Geometry check sheet. Reference: the model listing, model coordinates, mm. Give positions to 0.01 mm unless a question says otherwise; leave off trailing zeros. Loops run counter-clockwise (first coordinate to the right, second up) from the corner with the lowest first, then second, coordinate; pieces in that order, holes last. Notation, with made-up numbers: (7, 74.25) -> (32, 74.25) arc R29 ccw to (32, 113.25) -> close; hole circle Ø6 at (-22.5, -20.5). An arc over 180 degrees is marked (long way). Write item = value, one per line. Start each with the question number.
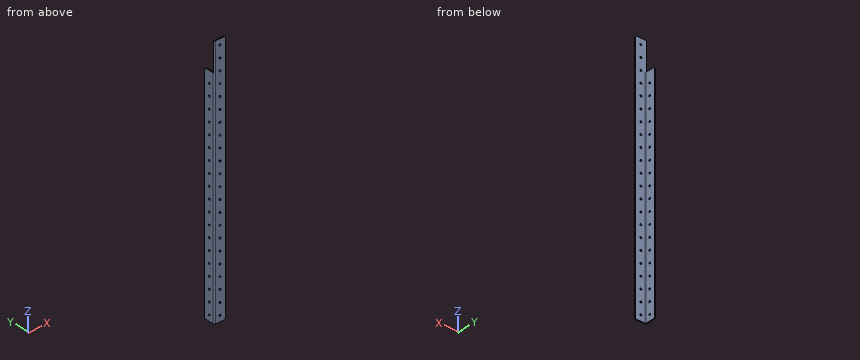
```python
from build123d import *

# Parameters (mm, degrees)
CUT_EXTRUDE1_OUTLINE_R   = 2.0701
CUT_EXTRUDE1_DEPTH       = 3.0988
CUT_EXTRUDE1_START       = 2.286
CUT_EXTRUDE1_2_OUTLINE_W = 2.286
CUT_EXTRUDE1_2_OUTLINE_H = 558.8
CUT_EXTRUDE1_2_DEPTH     = 23.114
CUT_EXTRUDE1_START_2     = 3.0988
CUT_EXTRUDE1_3_OUTLINE_W = 0.8128
CUT_EXTRUDE1_3_OUTLINE_H = 558.8
CUT_EXTRUDE1_3_DEPTH     = 22.3012
CUT_EXTRUDE1_4_OUTLINE_R = 2.0701
CUT_EXTRUDE1_4_DEPTH     = 2.286
CUT_EXTRUDE1_START_3     = -749.3
CUT_EXTRUDE1_5_DEPTH     = 558.8
CUT_EXTRUDE1_START_4     = 546.268979845
CUT_EXTRUDE1_6_OUTLINE_W = 4
CUT_EXTRUDE1_6_OUTLINE_H = 359
CUT_EXTRUDE1_6_DEPTH     = 2.731020155
CHAMFER1_SIZE            = 2.159
CUT_EXTRUDE2_START       = -2.286
SKETCH2_W                = 63.5
SKETCH2_H                = 23.114
CUT_EXTRUDE2_DEPTH       = 3.0988
CHAMFER2_SIZE            = 2.159
BOSS_EXTRUDE1_START      = -2.286
BOSS_EXTRUDE1_DEPTH      = 2.286


with BuildPart() as part:
    # Cut-Extrude1: read off the stored shape, not the designer's step
    # Cut-Extrude1 outline → Cut-Extrude1 (new body)
    with BuildSketch(Plane(origin=(0, 0, 0), x_dir=(1, 0, 0), z_dir=(0, 1, 0))):
        Polygon((0, 749.3), (0, 190.5), (25.4, 190.5), (25.4, 747.141), (23.241, 749.3), align=None)
        with Locations((12.7, 736.6)):
            Circle(CUT_EXTRUDE1_OUTLINE_R, mode=Mode.SUBTRACT)
        with Locations((12.7, 203.2)):
            Circle(CUT_EXTRUDE1_OUTLINE_R, mode=Mode.SUBTRACT)
        with Locations((12.7, 228.6)):
            Circle(CUT_EXTRUDE1_OUTLINE_R, mode=Mode.SUBTRACT)
        with Locations((12.7, 254)):
            Circle(CUT_EXTRUDE1_OUTLINE_R, mode=Mode.SUBTRACT)
        with Locations((12.7, 279.4)):
            Circle(CUT_EXTRUDE1_OUTLINE_R, mode=Mode.SUBTRACT)
        with Locations((12.7, 304.8)):
            Circle(CUT_EXTRUDE1_OUTLINE_R, mode=Mode.SUBTRACT)
        with Locations((12.7, 330.2)):
            Circle(CUT_EXTRUDE1_OUTLINE_R, mode=Mode.SUBTRACT)
        with Locations((12.7, 355.6)):
            Circle(CUT_EXTRUDE1_OUTLINE_R, mode=Mode.SUBTRACT)
        with Locations((12.7, 381)):
            Circle(CUT_EXTRUDE1_OUTLINE_R, mode=Mode.SUBTRACT)
        with Locations((12.7, 406.4)):
            Circle(CUT_EXTRUDE1_OUTLINE_R, mode=Mode.SUBTRACT)
        with Locations((12.7, 431.8)):
            Circle(CUT_EXTRUDE1_OUTLINE_R, mode=Mode.SUBTRACT)
        with Locations((12.7, 457.2)):
            Circle(CUT_EXTRUDE1_OUTLINE_R, mode=Mode.SUBTRACT)
        with Locations((12.7, 482.6)):
            Circle(CUT_EXTRUDE1_OUTLINE_R, mode=Mode.SUBTRACT)
        with Locations((12.7, 508)):
            Circle(CUT_EXTRUDE1_OUTLINE_R, mode=Mode.SUBTRACT)
        with Locations((12.7, 533.4)):
            Circle(CUT_EXTRUDE1_OUTLINE_R, mode=Mode.SUBTRACT)
        with Locations((12.7, 558.8)):
            Circle(CUT_EXTRUDE1_OUTLINE_R, mode=Mode.SUBTRACT)
        with Locations((12.7, 584.2)):
            Circle(CUT_EXTRUDE1_OUTLINE_R, mode=Mode.SUBTRACT)
        with Locations((12.7, 609.6)):
            Circle(CUT_EXTRUDE1_OUTLINE_R, mode=Mode.SUBTRACT)
        with Locations((12.7, 635)):
            Circle(CUT_EXTRUDE1_OUTLINE_R, mode=Mode.SUBTRACT)
        with Locations((12.7, 660.4)):
            Circle(CUT_EXTRUDE1_OUTLINE_R, mode=Mode.SUBTRACT)
        with Locations((12.7, 685.8)):
            Circle(CUT_EXTRUDE1_OUTLINE_R, mode=Mode.SUBTRACT)
        with Locations((12.7, 711.2)):
            Circle(CUT_EXTRUDE1_OUTLINE_R, mode=Mode.SUBTRACT)
    extrude(amount=CUT_EXTRUDE1_DEPTH)

    # Cut-Extrude1 2 outline → Cut-Extrude1 2 (add)
    with BuildSketch(Plane(origin=(0, 0, 0), x_dir=(1, 0, 0), z_dir=(0, 1, 0)).offset(CUT_EXTRUDE1_START)):
        with Locations((1.143, 469.9)):
            Rectangle(CUT_EXTRUDE1_2_OUTLINE_W, CUT_EXTRUDE1_2_OUTLINE_H)
    extrude(amount=CUT_EXTRUDE1_2_DEPTH)

    # Cut-Extrude1 3 outline → Cut-Extrude1 3 (cut)
    with BuildSketch(Plane.YZ.offset(CUT_EXTRUDE1_START_2)):
        with Locations((2.6924, -469.9)):
            Rectangle(CUT_EXTRUDE1_3_OUTLINE_W, CUT_EXTRUDE1_3_OUTLINE_H)
    extrude(amount=CUT_EXTRUDE1_3_DEPTH, mode=Mode.SUBTRACT)

    # Cut-Extrude1 4 outline → Cut-Extrude1 4 (cut)
    with BuildSketch(Plane.YZ):
        with Locations((12.7, -736.6)):
            Circle(CUT_EXTRUDE1_4_OUTLINE_R)
        with Locations((12.7, -711.2)):
            Circle(CUT_EXTRUDE1_4_OUTLINE_R)
        with Locations((12.7, -685.8)):
            Circle(CUT_EXTRUDE1_4_OUTLINE_R)
        with Locations((12.7, -660.4)):
            Circle(CUT_EXTRUDE1_4_OUTLINE_R)
        with Locations((12.7, -635)):
            Circle(CUT_EXTRUDE1_4_OUTLINE_R)
        with Locations((12.7, -609.6)):
            Circle(CUT_EXTRUDE1_4_OUTLINE_R)
        with Locations((12.7, -584.2)):
            Circle(CUT_EXTRUDE1_4_OUTLINE_R)
        with Locations((12.7, -558.8)):
            Circle(CUT_EXTRUDE1_4_OUTLINE_R)
        with Locations((12.7, -533.4)):
            Circle(CUT_EXTRUDE1_4_OUTLINE_R)
        with Locations((12.7, -508)):
            Circle(CUT_EXTRUDE1_4_OUTLINE_R)
        with Locations((12.7, -482.6)):
            Circle(CUT_EXTRUDE1_4_OUTLINE_R)
        with Locations((12.7, -457.2)):
            Circle(CUT_EXTRUDE1_4_OUTLINE_R)
        with Locations((12.7, -431.8)):
            Circle(CUT_EXTRUDE1_4_OUTLINE_R)
        with Locations((12.7, -406.4)):
            Circle(CUT_EXTRUDE1_4_OUTLINE_R)
        with Locations((12.7, -381)):
            Circle(CUT_EXTRUDE1_4_OUTLINE_R)
        with Locations((12.7, -355.6)):
            Circle(CUT_EXTRUDE1_4_OUTLINE_R)
        with Locations((12.7, -330.2)):
            Circle(CUT_EXTRUDE1_4_OUTLINE_R)
        with Locations((12.7, -304.8)):
            Circle(CUT_EXTRUDE1_4_OUTLINE_R)
        with Locations((12.7, -279.4)):
            Circle(CUT_EXTRUDE1_4_OUTLINE_R)
        with Locations((12.7, -254)):
            Circle(CUT_EXTRUDE1_4_OUTLINE_R)
        with Locations((12.7, -228.6)):
            Circle(CUT_EXTRUDE1_4_OUTLINE_R)
        with Locations((12.7, -203.2)):
            Circle(CUT_EXTRUDE1_4_OUTLINE_R)
    extrude(amount=CUT_EXTRUDE1_4_DEPTH, mode=Mode.SUBTRACT)

    # Cut-Extrude1 5 outline → Cut-Extrude1 5 (cut)
    with BuildSketch(Plane.XY.offset(CUT_EXTRUDE1_START_3)):
        with BuildLine():
            ThreePointArc((3.0988, 0), (0.907617506, 0.907617506), (0, 3.0988))
            Line((0, 3.0988), (0, 0))
            Line((0, 0), (3.0988, 0))
        make_face()
        with BuildLine():
            Line((3.0988, 3.0988), (2.286, 3.0988))
            ThreePointArc((2.286, 3.0988), (2.524063608, 2.524063608), (3.0988, 2.286))
            Line((3.0988, 2.286), (3.0988, 3.0988))
        make_face()
    extrude(amount=CUT_EXTRUDE1_5_DEPTH, mode=Mode.SUBTRACT)

    # Cut-Extrude1 6 outline → Cut-Extrude1 6 (cut)
    with BuildSketch(Plane(origin=(0, 0, 0), x_dir=(1, 0, 0), z_dir=(0, 0.7071067811865511, -0.7071067811865441)).offset(CUT_EXTRUDE1_START_4)):
        with Locations((2, 349.5)):
            Rectangle(CUT_EXTRUDE1_6_OUTLINE_W, CUT_EXTRUDE1_6_OUTLINE_H)
    extrude(amount=CUT_EXTRUDE1_6_DEPTH, mode=Mode.SUBTRACT)

    # Chamfer1
    chamfer1_edges = [part.edges().sort_by_distance(p)[0] for p in [
        (1.143, 25.4, -190.5),
        (25.4, 1.143, -190.5),
    ]]
    chamfer(chamfer1_edges, length=CHAMFER1_SIZE)

    # Sketch2 → Cut-Extrude2 (cut)
    with BuildSketch(Plane(origin=(2.286, 0, 0), x_dir=(0, 0, -1), z_dir=(1, 0, 0)).offset(CUT_EXTRUDE2_START)):
        with Locations((222.25, 13.843)):
            Rectangle(SKETCH2_W, SKETCH2_H)
    extrude(amount=CUT_EXTRUDE2_DEPTH, mode=Mode.SUBTRACT)

    # Chamfer2
    chamfer2_edges = [part.edges().sort_by_distance(p)[0] for p in [
        (1.143, 25.4, -254),
    ]]
    chamfer(chamfer2_edges, length=CHAMFER2_SIZE)

    # Sketch3 → Boss-Extrude1 (add)
    with BuildSketch(Plane(origin=(2.286, 0, 0), x_dir=(0, 0, -1), z_dir=(1, 0, 0)).offset(BOSS_EXTRUDE1_START)):
        with BuildLine():
            Line((254, 10.6299), (254, 14.7701))
            ThreePointArc((254, 14.7701), (256.0701, 12.7), (254, 10.6299))
        make_face()
    extrude(amount=BOSS_EXTRUDE1_DEPTH)


solid = part.part
```
1) Depth check by flat-ended pin: pin 1 Ø5 at (x, z) = (12.7, -482.6) entering from +Y; pin 2 Ø3 at (y, z) = (18, -626) entering from -X; pin 3 Ø8 at (y, z) = (13.5, -647) entering from +X; pin 4 Ø4 at (x, y) = (3.5, 11.5) entering from +Z. Enter the tip coordinate at first touch or a pass-through.
2) Section check A-A (z = -702). Enter the section's corners in (x, y).
3) Thickness scan on line 1 (Y direction, x = 5, z = -533.5); line 2 (Y direction, x = 1.55, z = -482.6). Record the ranges inside material, lowest first.
Check result:
q1.pin_1 = 2.29
q1.pin_2 = 0
q1.pin_3 = 2.29
q1.pin_4 = -254
q2.outline = (0, 3.1) arc R3.1 ccw to (3.1, 0) -> (25.4, 0) -> (25.4, 2.29) -> (3.1, 2.29) arc R0.81 cw to (2.29, 3.1) -> (2.29, 25.4) -> (0, 25.4) -> close
q3.line_1 = 0 to 2.29
q3.line_2 = 0.41 to 10.63, 14.77 to 25.4
